from build123d import *

# Parameters (mm, degrees)
F0_W     = 200
F0_H     = 49
F0_R     = 2.625
F1_DEPTH = 1.6
F3_W     = 200
F3_H     = 1.6
F4_DEPTH = 45
F5_R     = 2


with BuildPart() as f1:
    # F0 (on Top) → F1 (new body)
    with BuildSketch(Plane.XY):
        with Locations((0, -1)):
            Rectangle(F0_W, F0_H)
        with Locations((60, -15)):
            Circle(F0_R, mode=Mode.SUBTRACT)
        with Locations((60, 15)):
            Circle(F0_R, mode=Mode.SUBTRACT)
    extrude(amount=-F1_DEPTH)

    # F3 (on face) → F4 (join)
    with BuildSketch(Plane(origin=(0, 0, -1.6), x_dir=(1, 0, 0), z_dir=(0, 0, -1))):
        with Locations((0, 24.7)):
            Rectangle(F3_W, F3_H)
    extrude(amount=F4_DEPTH)

    # F5
    f5_edges = [f1.edges().sort_by_distance(p)[0] for p in [
        (0, -23.9, -1.6),
        (0, -25.5, 0),
    ]]
    fillet(f5_edges, radius=F5_R)


solid = f1.part
Work out the finished part from the listing and answer in its coordinate system (mm). A direction names the side the tool comes from. Coordinates: 2 decimals unless noted, no trailing zeros. Order: outer loops, then holes, each group sorted by start corner. A loop starts at its lowest first (then second) coordinate and runs counter-clockwise, first axis right, second up. Notation, with made-up numbers: (-33, 44.25) - (-10, 44.25) arc R21 cw to (-10, 82.25) - close; hole circle Ø6 at (41.25, -30.75). An arc over 180 degrees is marked (long way). Put each result on its own line as item: value. Start each with the question number.
1) Find section C-C (x = -47). Give the vertices of the cut face in (y, z), plus the area to 3 significant figures.
2) Find section D-D (z = -34). Give the vertices of the cut face in (x, y).
3) Find section A-A (y = -15). Give the vertices of the cut face in (x, z) (3 decimals), plus the area to 3 significant figures.
4) For a pull along Y with two mould halves and no side action, classify faces 1 (the flat face through (-1, -23.9, -25)), 2 (the cylindrical face through (62.5, -14.2, -0.8)), 3 (the cylindrical face through (62.5, 15.8, -0.8)), 4 (the flat face through (-100, -12, -1)) as released by +Y, released by -Y, zero draft, split by the parting line, or undercut.
5) Flat-ended cylindrical pins translate along their axes: pin 1 (6 mm diameter, centred on x = -7.5, y = -2, fed in from -Z); pin 2 (7 mm diameter, centred on x = 60, y = -15, fed in from +Z); pin 3 (3 mm diameter, centred on x = 60, y = 15, fed in from -Z); pin 4 (5 mm diameter, centred on x = 58, z = -22, fed in from +Y). Find the tip coordinate at first contact, or state that the pin passes through.
6) Find the intervals of material crossed by line 1 (Y direction, x = 60, z = -0.85) (3 decimals); line 2 (Y direction, x = 60, z = -1) (3 decimals); line 3 (Z direction, x = -77, y = 15), in increasing order. Write a range as from..to.
7) Find section B-B (x = 60). Give the vertices of the cut face in (y, z) (3 decimals).
8) For faces 5 (the flat face through (100, -12, -1)), 6 (the flat face through (-1, 1, -1.6)), determine the directions among +Z, -Z, +X, -X, +Y, -Y from which every point of the face is accessible in a straight line to the end or side of a thin tool.
Results list:
1. outline: (-25.5, -46.6) - (-23.9, -46.6) - (-23.9, -3.6) arc R2 cw to (-21.9, -1.6) - (23.5, -1.6) - (23.5, 0) - (-23.5, 0) arc R2 ccw to (-25.5, -2) - close
1. area: 150 mm^2
2. outline: (-100, -25.5) - (100, -25.5) - (100, -23.9) - (-100, -23.9) - close
3. outline: (-100, -1.6) - (57.375, -1.6) - (57.375, 0) - (-100, 0) - close; (62.625, -1.6) - (100, -1.6) - (100, 0) - (62.625, 0) - close
3. area: 312 mm^2
4. face 1: released by +Y
4. face 2: undercut
4. face 3: undercut
4. face 4: zero draft
5. pin 1: stops at z = -1.6
5. pin 2: stops at z = 0
5. pin 3: passes through
5. pin 4: stops at y = -23.9
6. line 1: y = -25.136..-17.625, -12.375..12.375, 17.625..23.5
6. line 2: y = -25.232..-17.625, -12.375..12.375, 17.625..23.5
6. line 3: z = -1.6..0
7. outline: (-25.5, -46.6) - (-23.9, -46.6) - (-23.9, -3.6) arc R2 cw to (-21.9, -1.6) - (-17.625, -1.6) - (-17.625, 0) - (-23.5, 0) arc R2 ccw to (-25.5, -2) - close; (-12.375, -1.6) - (12.375, -1.6) - (12.375, 0) - (-12.375, 0) - close; (17.625, -1.6) - (23.5, -1.6) - (23.5, 0) - (17.625, 0) - close
8. face 5: +Z, -Z, +X, +Y, -Y
8. face 6: -Z, +X, -X, +Y
